Verification items for the finished model (mm, model axes). Face numbers are marked on the shaded views. A direction names the side the tool comes from. Coordinates: 2 decimals unless noted, no trailing zeros. Order: outer loops, then holes, each group sorted by start corner. A loop starts at its lowest first (then second) coordinate and runs counter-clockwise, first axis right, second up. Notation, with made-up numbers: M -26,58.25 L 31,58.25 A21 cw 31,89.25 Z; hole C 50,23.5 d3. An arc over 180 degrees is marked long. Answer as a JSON object with one key per item and string values. Group by question number.
(1) Cross-section at B-B (z = 1.25). Enter the section's corners in (x, y), plus the area to 3 significant figures.
(2) Material ranges on line 1 (Y direction, x = 0, z = 7.3); line 2 (X direction, y = 5, z = 2.9); line 3 (Y direction, x = 0, z = 3.7), recorded low to high.
(3) Cross-section at D-D (y = -9.5). Enter the section's corners in (x, z).
(4) Cross-section at C-C (y = 5). Enter the section's corners in (x, z), plus the area to 3 significant figures.
(5) Access from +Z, -Z, +X, -X, +Y, -Y to the whole of each face (thin tool, end or side, straight path). Record for the marked faces 4 and 5.
(6) Gauge pin test, flat ends, axial feed: pin 1 Ø1.5 at (x, y) = (-3, -15) entering from +Z; pin 2 Ø2.5 at (x, y) = (-0.5, -4) entering from +Z; pin 3 Ø4 at (x, y) = (0, 5) entering from -Z. Record the tip position at first contact, or that the pin passes through.
(7) Mould release check, pull along Y, two halves, no side actions. Record for the marked faces 1, 2 and 3: released by +Y, released by -Y, zero draft, split by the parting line, or undercut.
(8) Cross-section at A-A (x = 0). Enter the section's corners in (y, z), plus the area to 3 significant figures.
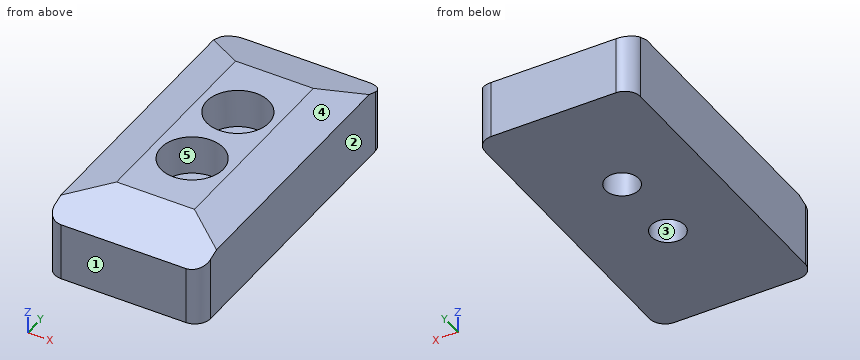
from build123d import *

# Parameters (mm, degrees)
SKETCH1_W           = 20
SKETCH1_H           = 40
SKETCH1_R           = 2.15
BOSS_EXTRUDE1_DEPTH = 10
CHAMFER1_SIZE       = 5
CHAMFER1_SIZE2      = 1.339745962
CHAMFER2_SIZE       = 7
CHAMFER2_SIZE2      = 2.54779164
SKETCH2_R           = 4
CUT_EXTRUDE1_DEPTH  = 5
FILLET1_R           = 2


with BuildPart() as part:
    # Sketch1 → Boss-Extrude1 (new body)
    with BuildSketch(Plane.XY):
        Rectangle(SKETCH1_W, SKETCH1_H)
        with Locations((0, -5)):
            Circle(SKETCH1_R, mode=Mode.SUBTRACT)
        with Locations((0, 5)):
            Circle(SKETCH1_R, mode=Mode.SUBTRACT)
    extrude(amount=BOSS_EXTRUDE1_DEPTH)

    # Chamfer1
    chamfer1_edges = [part.edges().sort_by_distance(p)[0] for p in [
        (-10, 0, 10),
        (10, 0, 10),
    ]]
    chamfer1_side = [part.faces().sort_by_distance(p)[0] for p in [
        (0, 0, 10),
    ]]
    chamfer(chamfer1_edges, length=CHAMFER1_SIZE, length2=CHAMFER1_SIZE2, reference=chamfer1_side[0])

    # Chamfer2
    chamfer2_edges = [part.edges().sort_by_distance(p)[0] for p in [
        (0, -20, 10),
        (0, 20, 10),
    ]]
    chamfer2_side = [part.faces().sort_by_distance(p)[0] for p in [
        (0, 0, 10),
    ]]
    chamfer(chamfer2_edges, length=CHAMFER2_SIZE, length2=CHAMFER2_SIZE2, reference=chamfer2_side[0])

    # Sketch2 → Cut-Extrude1 (cut)
    with BuildSketch(Plane.XY.offset(10)):
        with Locations((0, 5)):
            Circle(SKETCH2_R)
        with Locations((0, -5)):
            Circle(SKETCH2_R)
    extrude(amount=-CUT_EXTRUDE1_DEPTH, mode=Mode.SUBTRACT)

    # Fillet1
    fillet1_edges = [part.edges().sort_by_distance(p)[0] for p in [
        (10, 20, 3.72610418),
        (10, -20, 3.72610418),
        (-10, -20, 3.72610418),
        (-10, 20, 3.72610418),
    ]]
    fillet(fillet1_edges, radius=FILLET1_R)


solid = part.part
Taken from the geometry:
{
 "1": {"outline": "M -10,-18 A2 ccw -8,-20 L 8,-20 A2 ccw 10,-18 L 10,18 A2 ccw 8,20 L -8,20 A2 ccw -10,18 Z; hole C 0,-5 d4.3; hole C 0,5 d4.3", "area": "768 mm²"},
 "2": {"line 1": "y = -20 to -9, -1 to 1, 9 to 20", "line 2": "x = -10 to -2.15, 2.15 to 10", "line 3": "y = -20 to -7.15, -2.85 to 2.85, 7.15 to 20"},
 "3": {"outline": "M -10,0 L 10,0 L 10,8.66 L 5,10 L -5,10 L -10,8.66 Z"},
 "4": {"outline": "M -10,0 L -2.15,0 L -2.15,5 L -4,5 L -4,10 L -5,10 L -10,8.66 Z; M 2.15,0 L 10,0 L 10,8.66 L 5,10 L 4,10 L 4,5 L 2.15,5 Z", "area": "132 mm²"},
 "5": {"face 4": "+Z, +X, +Y, -Y", "face 5": "+Z"},
 "6": {"pin 1": "stops at z = 9.55", "pin 2": "stops at z = 5", "pin 3": "passes through"},
 "7": {"face 1": "released by -Y", "face 2": "zero draft", "face 3": "undercut"},
 "8": {"outline": "M -20,0 L -7.15,0 L -7.15,5 L -9,5 L -9,10 L -13,10 L -20,7.45 Z; M -2.85,0 L 2.85,0 L 2.85,5 L 1,5 L 1,10 L -1,10 L -1,5 L -2.85,5 Z; M 7.15,0 L 20,0 L 20,7.45 L 13,10 L 9,10 L 9,5 L 7.15,5 Z", "area": "259 mm²"}
}
